Design review of the part built by this model. Coordinates are the model's own, in mm. A direction names the side the tool comes from. Round coordinates to 2 decimals unless told otherwise and drop trailing zeros. Write each loop counter-clockwise with the first axis right and the second up, starting at its lowest first coordinate (ties: lowest second). Pieces come first, ordered by that corner, then holes.
from build123d import *

# Parameters (mm, degrees)
SKETCH1_W           = 600
SKETCH1_H           = 200
BOSS_EXTRUDE1_DEPTH = 5
SKETCH2_W           = 590
SKETCH2_H           = 70
BOSS_EXTRUDE2_DEPTH = 17.5
SKETCH3_R           = 1
CUT_EXTRUDE1_DEPTH  = 5


with BuildPart() as part:
    # Sketch1 → Boss-Extrude1 (new body)
    with BuildSketch(Plane(origin=(0, 0, 0), x_dir=(1, 0, 0), z_dir=(0, 1, 0))):
        with Locations((300, 100)):
            Rectangle(SKETCH1_W, SKETCH1_H)
    extrude(amount=BOSS_EXTRUDE1_DEPTH)

    # Sketch2 → Boss-Extrude2 (add)
    with BuildSketch(Plane(origin=(0, 5, 0), x_dir=(1, 0, 0), z_dir=(0, 1, 0))):
        Polygon((0, 200), (5, 200), (595, 200), (600, 200), (600, 0), (595, 0), (595, 120), (5, 120), (5, 0), (0, 0), align=None)
        with Locations((300, 160)):
            Rectangle(SKETCH2_W, SKETCH2_H, mode=Mode.SUBTRACT)
    extrude(amount=BOSS_EXTRUDE2_DEPTH)

    # Sketch3 → Cut-Extrude1 (cut)
    with BuildSketch(Plane.XY.offset(-120)):
        with Locations((21, 13.75)):
            Circle(SKETCH3_R)
        with Locations((37, 13.75)):
            Circle(SKETCH3_R)
        with Locations((53, 13.75)):
            Circle(SKETCH3_R)
        with Locations((69, 13.75)):
            Circle(SKETCH3_R)
        with Locations((85, 13.75)):
            Circle(SKETCH3_R)
        with Locations((101, 13.75)):
            Circle(SKETCH3_R)
        with Locations((117, 13.75)):
            Circle(SKETCH3_R)
        with Locations((133, 13.75)):
            Circle(SKETCH3_R)
        with Locations((149, 13.75)):
            Circle(SKETCH3_R)
        with Locations((165, 13.75)):
            Circle(SKETCH3_R)
        with Locations((181, 13.75)):
            Circle(SKETCH3_R)
        with Locations((197, 13.75)):
            Circle(SKETCH3_R)
        with Locations((213, 13.75)):
            Circle(SKETCH3_R)
        with Locations((229, 13.75)):
            Circle(SKETCH3_R)
        with Locations((245, 13.75)):
            Circle(SKETCH3_R)
        with Locations((261, 13.75)):
            Circle(SKETCH3_R)
        with Locations((277, 13.75)):
            Circle(SKETCH3_R)
        with Locations((293, 13.75)):
            Circle(SKETCH3_R)
        with Locations((309, 13.75)):
            Circle(SKETCH3_R)
        with Locations((325, 13.75)):
            Circle(SKETCH3_R)
        with Locations((341, 13.75)):
            Circle(SKETCH3_R)
        with Locations((357, 13.75)):
            Circle(SKETCH3_R)
        with Locations((373, 13.75)):
            Circle(SKETCH3_R)
        with Locations((389, 13.75)):
            Circle(SKETCH3_R)
        with Locations((405, 13.75)):
            Circle(SKETCH3_R)
        with Locations((421, 13.75)):
            Circle(SKETCH3_R)
        with Locations((437, 13.75)):
            Circle(SKETCH3_R)
        with Locations((453, 13.75)):
            Circle(SKETCH3_R)
        with Locations((469, 13.75)):
            Circle(SKETCH3_R)
        with Locations((485, 13.75)):
            Circle(SKETCH3_R)
        with Locations((501, 13.75)):
            Circle(SKETCH3_R)
        with Locations((517, 13.75)):
            Circle(SKETCH3_R)
        with Locations((533, 13.75)):
            Circle(SKETCH3_R)
        with Locations((549, 13.75)):
            Circle(SKETCH3_R)
        with Locations((565, 13.75)):
            Circle(SKETCH3_R)
        with Locations((581, 13.75)):
            Circle(SKETCH3_R)
    extrude(amount=-CUT_EXTRUDE1_DEPTH, mode=Mode.SUBTRACT)


solid = part.part
1) The part is to be moulded in two halves that separate along X. For faces 4 (the face through (296, 0, -101)), 5 (the face through (5, 14, -61)), 6 (the face through (600, 11, -101)), say which applies: pulls with the +X half, pulls with the -X half, needs draft (parallel to the pull), parting line crosses it, or undercut.
2) Add section B-B on y = 9. State the section outline as (x, z) points.
3) Add section C-C on z = -145. State the section outline as (x, y) points, and give its area (4 significant figures).
4) For P1, Ø2.5, axis at x = 533, y = 13.75, coming from the +Z side; P2, Ø1.5, axis at x = 91.5, z = -104.5, coming from the +Y side; P3, Ø1.8, axis at x = 309, y = 13.75, coming from the +Z side, all flat-tipped, find the tip position at first contact; note any pin that passes through.
5) For faces 1 (the face through (296, 5, -61)), 2 (the face through (296, 14, -125)), 3 (the face through (304, 11, -200)), list the 3-axis set-ups (+Z, -Z, +X, -X, +Y, -Y) from which the entire face can be reached by the end or side of a thin tool; tool diameter is ignored.
6) Add section A-A on x = 493. State the section outline as (y, z) points.
7) For line 1 along Y through (x, z) = (309, -122.6); line 2 along X through (y, z) = (15, -144.5); line 3 along Z through (x, y) = (431.5, 14.25), list the stretches that pass through material, from the lowest coordinate up.
Computed:
1. face 4: needs draft
1. face 5: undercut
1. face 6: pulls with the +X half
2. outline: (0, -200) - (600, -200) - (600, 0) - (595, 0) - (595, -120) - (5, -120) - (5, 0) - (0, 0) - close; hole (5, -195) - (595, -195) - (595, -125) - (5, -125) - close
3. outline: (0, 0) - (600, 0) - (600, 22.5) - (595, 22.5) - (595, 5) - (5, 5) - (5, 22.5) - (0, 22.5) - close
3. area: 3,175 mm2
4. P1: stops at z = -120
4. P2: stops at y = 5
4. P3: stops at z = -195
5. face 1: +Z, +Y
5. face 2: +Y
5. face 3: -Z, +X, -X, +Y, -Y
6. outline: (0, -200) - (22.5, -200) - (22.5, -195) - (5, -195) - (5, -125) - (22.5, -125) - (22.5, -120) - (5, -120) - (5, 0) - (0, 0) - close
7. line 1: y = 0 to 12.75, 14.75 to 22.5
7. line 2: x = 0 to 5, 595 to 600
7. line 3: z = -200 to -195, -125 to -120
